```python
from build123d import *

# Parameters (mm, degrees)
F0_W           = 19.05
F0_H           = 19.05
F1_DEPTH       = 479.425
F3_D           = 6.35
F3_DEPTH       = 25.4
F3_CSINK_D     = 7.62
F3_CSINK_ANGLE = 90
F3_TIP         = 1.9077324654
F5_D           = 6.35
F5_DEPTH       = 25.4
F5_CSINK_D     = 7.62
F5_CSINK_ANGLE = 90
F5_TIP         = 1.9077324654
F6_R           = 2.54


with BuildPart() as f1:
    # F0 (on Right) → F1 (new body, symmetric)
    with BuildSketch(Plane.YZ):
        with Locations((-9.525, 9.525)):
            Rectangle(F0_W, F0_H)
    extrude(amount=F1_DEPTH, both=True)

    # F3
    with Locations(Plane(origin=(-479.425, 0, 0), x_dir=(0, -1, 0), z_dir=(-1, 0, 0))):
        with Locations((9.525, 9.525)):
            CounterSinkHole(F3_D / 2, F3_CSINK_D / 2, depth=F3_DEPTH, counter_sink_angle=F3_CSINK_ANGLE)
            with Locations((0, 0, -(F3_DEPTH + F3_TIP / 2))):  # 118° drill point
                Cone(0, F3_D / 2, F3_TIP, mode=Mode.SUBTRACT)

    # F5
    with Locations(Plane.YZ.offset(479.425)):
        with Locations((-9.525, 9.525)):
            CounterSinkHole(F5_D / 2, F5_CSINK_D / 2, depth=F5_DEPTH, counter_sink_angle=F5_CSINK_ANGLE)
            with Locations((0, 0, -(F5_DEPTH + F5_TIP / 2))):  # 118° drill point
                Cone(0, F5_D / 2, F5_TIP, mode=Mode.SUBTRACT)

    # F6
    f6_edges = [f1.edges().sort_by_distance(p)[0] for p in [
        (0, -19.05, 19.05),
        (0, -19.05, 0),
        (0, 0, 0),
        (0, 0, 19.05),
    ]]
    fillet(f6_edges, radius=F6_R)


solid = f1.part
```
Work out the finished part from the listing and answer in its coordinate system (mm). Coordinates: 2 decimals unless noted, no trailing zeros. Write each loop counter-clockwise with the first axis right and the second up, starting at its lowest first coordinate (ties: lowest second). Pieces come first, ordered by that corner, then holes.
Q1. Find the intervals of material crossed by line 1 (X direction, y = -12.25, z = 7.75); line 2 (X direction, y = -9, z = 13.25); line 3 (Z direction, x = 11, y = -1.25), in increasing order.
Q2. This flat-tipped pin is pushed along its axis until it touches: pin 1 Ø5 at (y, z) = (-9.525, 9.525) entering from +X. Where does it stop, or does it pass through?
Q3. A cutting plane is placed at A-A, the plane x = 54.5. Give the vertices of the cut face in (y, z).
Findings below:
1. line 1: x = -478.87 to 478.87
1. line 2: x = -479.38 to 479.38
1. line 3: z = 0.35 to 18.7
2. pin 1: stops at x = 453.62
3. outline: (-19.05, 2.54) arc R2.54 ccw to (-16.51, 0) - (-2.54, 0) arc R2.54 ccw to (0, 2.54) - (0, 16.51) arc R2.54 ccw to (-2.54, 19.05) - (-16.51, 19.05) arc R2.54 ccw to (-19.05, 16.51) - close
